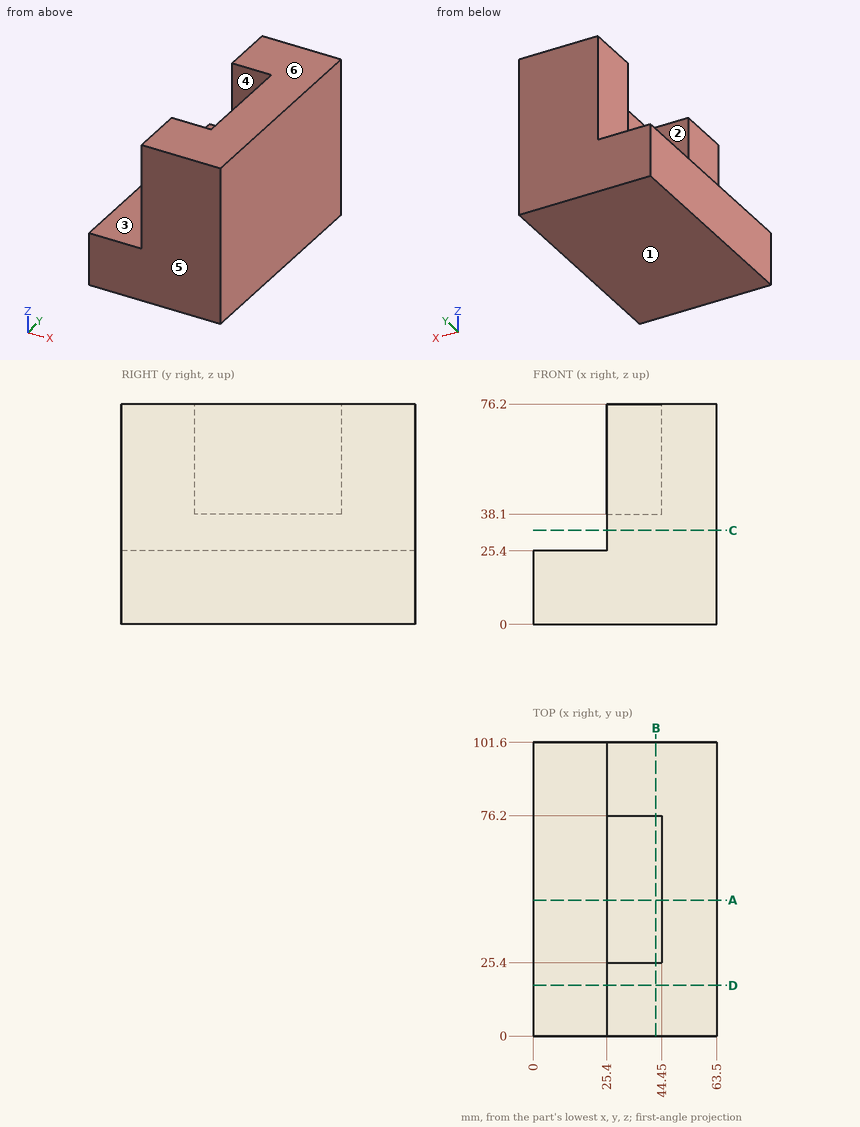
The figure shows three views and two pictorial views of one solid part (mm, origin at its lowest corner). Answer the questions. A direction names the side the tool comes from. Round coordinates to 2 decimals unless told otherwise and drop trailing zeros. Order: outer loops, then holes, each group sorted by start corner. A loop starts at its lowest first (then second) coordinate and runs counter-clockwise, first axis right, second up. Notation, with made-up numbers: (-17.75, 30.5) -> (9.25, 30.5) arc R21 cw to (9.25, 42.5) -> close; hole circle Ø8 at (50, -33.75). An arc over 180 degrees is marked (long way). Put each result on its own line as item: value.
Q1. Section D-D, the plane y = 17.5 is taken. Write down the section's boundary in (x, z), and give its area (3 significant figures).
Results list:
outline: (0, 0) -> (63.5, 0) -> (63.5, 76.2) -> (25.4, 76.2) -> (25.4, 25.4) -> (0, 25.4) -> close
area: 3,550 mm^2
Q2. Consider line 1 along Y through (x, z) = (36, 62); line 2 along X through (y, z) = (82, 65); line 3 along Z through (x, y) = (18, 40.5). Determine where each line is inside the solid, lowest interval first.
Results list:
line 1: 0 to 25.4, 76.2 to 101.6
line 2: 25.4 to 63.5
line 3: 0 to 25.4
Q3. Which of the six approach directions +Z, -Z, +X, -X, +Y, -Y give full straight-line access (tool end or side, diameter ignored) to the marked faces 1, 2 and 3?
Results list:
face 1: -Z, +X, -X, +Y, -Y
face 2: +Z, -X
face 3: +Z, -X, +Y, -Y
Q4. Each of these flat-tipped pins is pushed along its axis until it touches: P1, Ø2, axis at x = 38, y = 58.5, coming from the +Z side; P2, Ø12.5, axis at x = 9, y = 64, coming from the +Z side; P3, Ø12, axis at x = 17, y = 12.5, coming from the -Z side; P4, Ø12, axis at y = 45.5, z = 60.5, coming from the -X side. Where does it stop, or does it pass through?
Results list:
P1: z = 38.1
P2: z = 25.4
P3: z = 0
P4: x = 44.45
Q5. Section A-A, the plane y = 47 is taken. Write down the section's boundary in (x, z).
Results list:
outline: (0, 0) -> (63.5, 0) -> (63.5, 76.2) -> (44.45, 76.2) -> (44.45, 38.1) -> (25.4, 38.1) -> (25.4, 25.4) -> (0, 25.4) -> close
Q6. Section B-B, the plane x = 42.5 is taken. Write down the section's boundary in (y, z).
Results list:
outline: (0, 0) -> (101.6, 0) -> (101.6, 76.2) -> (76.2, 76.2) -> (76.2, 38.1) -> (25.4, 38.1) -> (25.4, 76.2) -> (0, 76.2) -> close
Q7. Determine the mould class of the marked faces 4, 5 and 6 for opening direction Y: pulls with the +Y half, pulls with the -Y half, needs draft (parallel to the pull), parting line crosses it, or undercut.
Results list:
face 4: undercut
face 5: pulls with the -Y half
face 6: needs draft
Q8. Section C-C, the plane z = 32.5 is taken. Write down the section's boundary in (x, y).
Results list:
outline: (25.4, 0) -> (63.5, 0) -> (63.5, 101.6) -> (25.4, 101.6) -> close
